```python
from build123d import *
from build123d.topology import SkipClean

# Parameters (mm, degrees)
SKETCH2_R           = 6
BOSS_EXTRUDE1_DEPTH = 16
SKETCH3_R           = 14
BOSS_EXTRUDE2_DEPTH = 40
SKETCH4_R           = 6
CUT_EXTRUDE1_DEPTH  = 56.948637328
SKETCH5_W           = 28
SKETCH5_H           = 30
BOSS_EXTRUDE3_DEPTH = 2.5
SKETCH8_R           = 15.28865651
SKETCH8_R_2         = 14
CUT_EXTRUDE2_DEPTH  = 35
SKETCH9_R           = 3
CUT_EXTRUDE3_DEPTH  = 35
CUT_EXTRUDE4_DEPTH  = 81.18883969
SKETCH11_W          = 30
SKETCH11_H          = 5
CUT_EXTRUDE5_DEPTH  = 15
SKETCH14_R          = 2.5
BOSS_EXTRUDE4_DEPTH = 15
SKETCH17_W          = 12
SKETCH17_H          = 12
BOSS_EXTRUDE6_DEPTH = 5


with BuildPart() as part:
    # Sketch2 → Boss-Extrude1 (new, symmetric)
    with BuildSketch(Plane(origin=(0, 0, 0), x_dir=(0, 0, -1), z_dir=(1, 0, 0))):
        with BuildLine():
            Line((-25, -17.5), (-4.873971328, -21.965755245))
            ThreePointArc((-4.873971328, -21.965755245), (22.5, 0), (-4.873971328, 21.965755245))
            Line((-4.873971328, 21.965755245), (-25, 17.5))
            Line((-25, 17.5), (-25, -17.5))
        make_face()
        Circle(SKETCH2_R, mode=Mode.SUBTRACT)
    extrude(amount=BOSS_EXTRUDE1_DEPTH, both=True)

    # Sketch3 → Boss-Extrude2 (add)
    with BuildSketch(Plane.XY):
        Circle(SKETCH3_R)
    extrude(amount=-BOSS_EXTRUDE2_DEPTH)

    # Sketch4 → Cut-Extrude1 (cut, through all)
    with BuildSketch(Plane(origin=(16, 0, 0), x_dir=(0, 0, -1), z_dir=(1, 0, 0))):
        Circle(SKETCH4_R)
    extrude(amount=-CUT_EXTRUDE1_DEPTH, mode=Mode.SUBTRACT)

    # Sketch5 → Boss-Extrude3 (add, symmetric)
    with BuildSketch(Plane(origin=(0, 0, 0), x_dir=(1, 0, 0), z_dir=(0, 1, 0))):
        with Locations((0, 55)):
            Rectangle(SKETCH5_W, SKETCH5_H)
    extrude(amount=BOSS_EXTRUDE3_DEPTH, both=True)

    # Sketch8 → Cut-Extrude2 (cut)
    with BuildSketch(Plane(origin=(0, 0, -70), x_dir=(-1, 0, 0), z_dir=(0, 0, -1))):
        Circle(SKETCH8_R)
        with Locations(Location((0, 0, 0), (0, 0, 180))):
            Circle(SKETCH8_R_2, mode=Mode.SUBTRACT)
    extrude(amount=-CUT_EXTRUDE2_DEPTH, mode=Mode.SUBTRACT)

    # Sketch9 → Cut-Extrude3 (cut)
    with BuildSketch(Plane(origin=(0, 2.5, 0), x_dir=(1, 0, 0), z_dir=(0, 1, 0))):
        with Locations(Location((-9, 62, 0), (0, 0, 270))):
            Circle(SKETCH9_R)
        with Locations(Location((9, 62, 0), (0, 0, 270))):
            Circle(SKETCH9_R)
    extrude(amount=-CUT_EXTRUDE3_DEPTH, mode=Mode.SUBTRACT)

    # Sketch10 → Cut-Extrude4 (cut, through all)
    with SkipClean():  # the faces are left unmerged after this step: merging them gives an invalid solid
        with BuildSketch(Plane(origin=(16, 0, 0), x_dir=(0, 0, -1), z_dir=(1, 0, 0))):
            with BuildLine():
                Line((-25, -17.5), (-4.873971328, -21.965755245))
                ThreePointArc((-4.873971328, -21.965755245), (-22.5, 0), (-4.873971328, 21.965755245))
                Line((-4.873971328, 21.965755245), (-25, 17.5))
                Line((-25, 17.5), (-25, -17.5))
            make_face()
        extrude(amount=-CUT_EXTRUDE4_DEPTH, mode=Mode.SUBTRACT)

    # Sketch11 → Cut-Extrude5 (cut, symmetric)
    with SkipClean():  # the faces are left unmerged after this step: merging them gives an invalid solid
        with BuildSketch(Plane(origin=(0, 0, 0), x_dir=(0, 0, -1), z_dir=(1, 0, 0))):
            with Locations((55, 0)):
                Rectangle(SKETCH11_W, SKETCH11_H)
        extrude(amount=CUT_EXTRUDE5_DEPTH, both=True, mode=Mode.SUBTRACT)

    # Sketch14 → Boss-Extrude4 (add)
    with SkipClean():  # the faces are left unmerged after this step: merging them gives an invalid solid
        with BuildSketch(Plane(origin=(0, 0, -40), x_dir=(-1, 0, 0), z_dir=(0, 0, -1))):
            Circle(SKETCH14_R)
        extrude(amount=BOSS_EXTRUDE4_DEPTH)

    # Sketch17 → Boss-Extrude6 (add)
    with SkipClean():  # the faces are left unmerged after this step: merging them gives an invalid solid
        with BuildSketch(Plane(origin=(0, 0, -40), x_dir=(-1, 0, 0), z_dir=(0, 0, -1))):
            Rectangle(SKETCH17_W, SKETCH17_H)
        extrude(amount=BOSS_EXTRUDE6_DEPTH)


solid = part.part
```
The listing builds one solid part. Answer for the finished solid, in the listing's coordinates (mm). A direction names the side the tool comes from. Coordinates: 2 decimals unless noted, no trailing zeros. Loops run counter-clockwise (first coordinate to the right, second up) from the corner with the lowest first, then second, coordinate; pieces in that order, holes last. Notation, with made-up numbers: M 23,68.25 L 57,68.25 A10 cw 57,73.25 Z; hole C 89,-23 d6. An arc over 180 degrees is marked long. Answer as CSV lines item,"result". Start each with the question number.
(1) The part is cut by section C-C (y = -8). Give the vertices of the cut face in (x, z), and give its area (3 significant figures).
(2) Given pin 1 (4 mm diameter, centred on y = -1, z = -41.5, fed in from +X); pin 2 (8 mm diameter, centred on y = -0.5, z = -34.5, fed in from -X); pin 3 (8 mm diameter, centred on x = 5, y = -14.5, fed in from +Z), each flat-ended and moving along its own axis, determine where each tip first touches the part or whether it passes through.
(3) For faces 3 (the flat face through (0, 6, -42)), 4 (the cylindrical face through (0.54, -2.44, -49.93)), 5 (the flat face through (6, 0, -42)), 6 (the flat face through (-6, 0, -42)), 7 (the flat face through (0, -6, -42)), determine the directions among +Z, -Z, +X, -X, +Y, -Y from which every point of the face is accessible in a straight line to the end or side of a thin tool.
(4) The part is cut by section B-B (z = -28.5). Give the vertices of the cut face in (x, y).
(5) The mould has two halves that part along Z. Classify faces 1 (the flat face through (0, 0, -55)), 2 (the cylindrical face through (-11.11, 8.52, -28.96)): pulls with the +Z half, pulls with the -Z half, needs draft (parallel to the pull), parting line crosses it, or undercut.
(6) The part is cut by section D-D (z = -14). Give the vertices of the cut face in (x, y).
(7) Find the intervals of material crossed by L1, parallel to Y at x = -10, z = 0; L2, parallel to Y at x = -13, z = 4; L3, parallel to Y at x = -3, z = -43, in increasing order. Write a range as [from, to].
(8) The part is cut by section A-A (x = 0). Give the vertices of the cut face in (y, z).
Determined:
1,outline,"M -16,-21.03 L -11.49,-21.03 L -11.49,-40 L 11.49,-40 L 11.49,-21.03 L 16,-21.03 L 16,21.03 L -16,21.03 Z"
1,area,"1,780 mm2"
2,pin 1,"x = 14"
2,pin 2,"x = -14"
2,pin 3,"z = 19.9"
3,face 3,"-Z, +X, -X, +Y"
3,face 4,"-Z"
3,face 5,"-Z, +X, +Y, -Y"
3,face 6,"-Z, -X, +Y, -Y"
3,face 7,"-Z, +X, -X, -Y"
4,outline,"C 0,0 d28"
5,face 1,"pulls with the -Z half"
5,face 2,"needs draft"
6,outline,"M -16,-17.61 L 16,-17.61 L 16,17.61 L -16,17.61 Z"
7,L1,"[-22.5, -6], [6, 22.5]"
7,L2,"[-22.14, -4.47], [4.47, 22.14]"
7,L3,"[-6, 6]"
8,outline,"M -14,-40 L -6,-40 L -6,-45 L -2.5,-45 L -2.5,-55 L 2.5,-55 L 2.5,-45 L 6,-45 L 6,-40 L 14,-40 L 14,-17.61 A22.5 ccw long -14,-17.61 Z; hole C 0,0 d12"
